The listing builds one solid part. Answer for the finished solid, in the listing's coordinates (mm). Face numbers are marked on the shaded views. Coordinates: 2 decimals unless noted, no trailing zeros. Write each loop counter-clockwise with the first axis right and the second up, starting at its lowest first coordinate (ties: lowest second). Pieces come first, ordered by that corner, then holes.
from build123d import *

# Parameters (mm, degrees)
SKETCH1_W           = 45
SKETCH1_H           = 62
BOSS_EXTRUDE1_DEPTH = 12
SKETCH2_R           = 7
SKETCH2_R_2         = 2.75
CUT_EXTRUDE1_DEPTH  = 12
SKETCH3_R           = 10
CUT_EXTRUDE2_DEPTH  = 2.5
SKETCH4_R           = 2
CUT_EXTRUDE3_DEPTH  = 16
SKETCH5_R           = 2
CUT_EXTRUDE4_DEPTH  = 16
CHAMFER1_SIZE       = 6


with BuildPart() as part:
    # Sketch1 → Boss-Extrude1 (new body)
    with BuildSketch(Plane(origin=(0, 0, 0), x_dir=(1, 0, 0), z_dir=(0, 1, 0))):
        Rectangle(SKETCH1_W, SKETCH1_H)
    extrude(amount=BOSS_EXTRUDE1_DEPTH)

    # Sketch2 → Cut-Extrude1 (cut)
    with BuildSketch(Plane(origin=(0, 12, 0), x_dir=(1, 0, 0), z_dir=(0, 1, 0))):
        with Locations((0, -18)):
            Circle(SKETCH2_R)
        with Locations((-18, 10.5)):
            Circle(SKETCH2_R_2)
        with Locations((18, 10.5)):
            Circle(SKETCH2_R_2)
    extrude(amount=-CUT_EXTRUDE1_DEPTH, mode=Mode.SUBTRACT)

    # Sketch3 → Cut-Extrude2 (cut)
    with BuildSketch(Plane(origin=(0, 12, 0), x_dir=(1, 0, 0), z_dir=(0, 1, 0))):
        with Locations((0, -18)):
            Circle(SKETCH3_R)
    extrude(amount=-CUT_EXTRUDE2_DEPTH, mode=Mode.SUBTRACT)

    # Sketch4 → Cut-Extrude3 (cut)
    with BuildSketch(Plane.ZY.offset(22.5)):
        with Locations((24, 6)):
            Circle(SKETCH4_R)
        with Locations((-3, 6)):
            Circle(SKETCH4_R)
    extrude(amount=-CUT_EXTRUDE3_DEPTH, mode=Mode.SUBTRACT)

    # Sketch5 → Cut-Extrude4 (cut)
    with BuildSketch(Plane(origin=(22.5, 0, 0), x_dir=(0, 0, -1), z_dir=(1, 0, 0))):
        with Locations((-24, 6)):
            Circle(SKETCH5_R)
        with Locations((3, 6)):
            Circle(SKETCH5_R)
    extrude(amount=-CUT_EXTRUDE4_DEPTH, mode=Mode.SUBTRACT)

    # Chamfer1
    chamfer1_edges = [part.edges().sort_by_distance(p)[0] for p in [
        (-22.5, 6, -31),
        (22.5, 6, -31),
    ]]
    chamfer(chamfer1_edges, length=CHAMFER1_SIZE)


solid = part.part
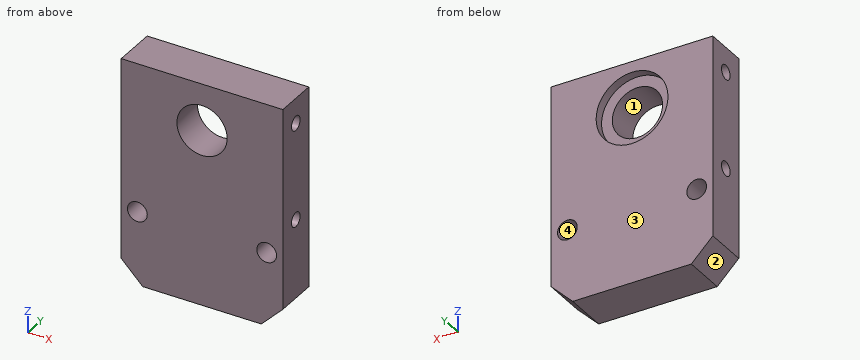
Q1. The part is cut by section B-B, the plane y = 1.5. Write down the section's boundary in (x, z).
Answers below:
outline: (-22.5, -25) - (-16.5, -31) - (16.5, -31) - (22.5, -25) - (22.5, 31) - (-22.5, 31) - close; hole circle Ø5.5 at (-18, -10.5); hole circle Ø14 at (0, 18); hole circle Ø5.5 at (18, -10.5)
Q2. Find the intervals of material crossed by probe 1 along X at (y, z) = (9, -10.5); probe 2 along Y at (x, z) = (15.25, 24); probe 3 along Z at (x, y) = (-10, 5.25), in increasing order.
Answers below:
probe 1: x = -22.5 to -20.75, -15.25 to 15.25, 20.75 to 22.5
probe 2: y = 0 to 4, 8 to 12
probe 3: z = -31 to -4.85, -1.15 to 22.15, 25.85 to 31
Q3. The part is cut by section D-D, the plane z = 24. Write down the section's boundary in (x, y), then the cut area to 3 significant figures.
Answers below:
outline: (-22.5, 0) - (-3.61, 0) - (-3.61, 9.5) - (-8, 9.5) - (-8, 12) - (-22.5, 12) - (-22.5, 8) - (-6.5, 8) - (-6.5, 4) - (-22.5, 4) - close; (3.61, 0) - (22.5, 0) - (22.5, 4) - (6.5, 4) - (6.5, 8) - (22.5, 8) - (22.5, 12) - (8, 12) - (8, 9.5) - (3.61, 9.5) - close
area: 303 mm2
Q4. The part is cut by section A-A, the plane x = -18. Write down the section's boundary in (y, z), then the cut area to 3 significant figures.
Answers below:
outline: (0, -29.5) - (12, -29.5) - (12, -13.25) - (0, -13.25) - close; (0, -7.75) - (12, -7.75) - (12, 31) - (0, 31) - close; hole circle Ø4 at (6, -3); hole circle Ø4 at (6, 24)
area: 635 mm2
Q5. Determine the mould class of the marked faces 1, 2, 3 and 4 for opening direction X: released by +X, released by -X, zero draft, split by the parting line, or undercut.
Answers below:
face 1: undercut
face 2: released by -X
face 3: zero draft
face 4: undercut
Q6. Given pin 1 (5 mm diameter, centred on y = 6, z = -3, fed in from +X); pin 2 (3.5 mm diameter, centred on y = 6, z = 24, fed in from +X); pin 3 (5 mm diameter, centred on x = -18, z = -10.5, fed in from +Y), each flat-ended and moving along its own axis, determine where each tip first touches the part or whether it passes through.
Answers below:
pin 1: stops at x = 22.5
pin 2: stops at x = 6.5
pin 3: passes through
Q7. The part is cut by section C-C, the plane x = 0. Write down the section's boundary in (y, z), then the cut area to 3 significant figures.
Answers below:
outline: (0, -31) - (12, -31) - (12, 8) - (9.5, 8) - (9.5, 11) - (0, 11) - close; (0, 25) - (9.5, 25) - (9.5, 28) - (12, 28) - (12, 31) - (0, 31) - close
area: 561 mm2
